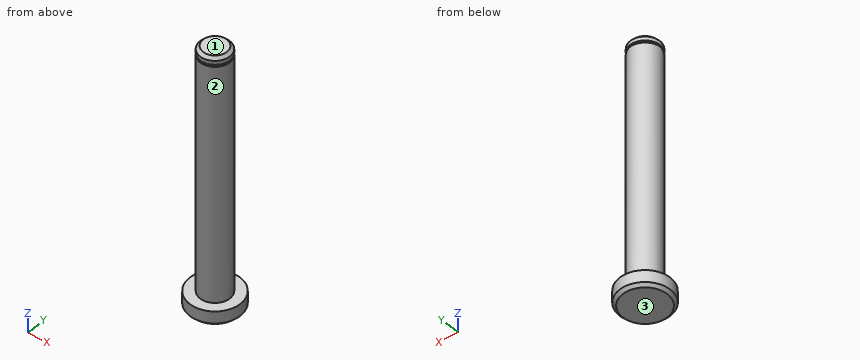
```python
from build123d import *

# Parameters (mm, degrees)
SKETCH1_R               = 8.5
BOSS_EXTRUDE1_DEPTH     = 5
SKETCH2_R               = 5
BOSS_EXTRUDE2_DEPTH     = 82
CHAMFER1_SIZE           = 1
SKETCH3_R               = 14.7
SKETCH3_R_2             = 4.7
CUT_EXTRUDE_THIN1_DEPTH = 0.7


with BuildPart() as part:
    # Sketch1 → Boss-Extrude1 (new body)
    with BuildSketch(Plane.XY):
        Circle(SKETCH1_R)
    extrude(amount=BOSS_EXTRUDE1_DEPTH)

    # Sketch2 → Boss-Extrude2 (add)
    with BuildSketch(Plane.XY.offset(5)):
        Circle(SKETCH2_R)
    extrude(amount=BOSS_EXTRUDE2_DEPTH)

    # Chamfer1
    chamfer1_edges = [part.edges().sort_by_distance(p)[0] for p in [
        (-8.5, 0, 0),
        (-5, 0, 87),
    ]]
    chamfer(chamfer1_edges, length=CHAMFER1_SIZE)

    # Sketch3 → Cut-Extrude-Thin1 (cut)
    with BuildSketch(Plane.XY.offset(84)):
        Circle(SKETCH3_R)
        Circle(SKETCH3_R_2, mode=Mode.SUBTRACT)
    extrude(amount=CUT_EXTRUDE_THIN1_DEPTH, mode=Mode.SUBTRACT)


solid = part.part
```
Source: CAD feature listing. Evaluate the final solid. Frame: model axes, mm. Face numbers are marked on the shaded views. Round coordinates to 2 decimals unless told otherwise and drop trailing zeros. Loops run counter-clockwise (first coordinate to the right, second up) from the corner with the lowest first, then second, coordinate; pieces in that order, holes last.
1. Contact query for flat-ended pins moving along their axis: pin 1 (1.5 mm diameter, centred on x = 1, z = 32, fed in from -Y); pin 2 (1 mm diameter, centred on y = 3, z = 23.5, fed in from +X); pin 3 (5 mm diameter, centred on x = -4, z = 56.5, fed in from +Y). Output: stop coordinate, or through.
2. Ray query, L1, parallel to Z at x = 1.5, y = -7; L2, parallel to Y at x = 1.75, z = 23; L3, parallel to X at y = 0.75, z = 38. Return the intervals inside material, ascending.
3. Section query A-A on x = 0. Output: boundary loops of the cut face in (y, z), and give its area (3 significant figures).
4. Section query C-C on z = 62. Output: boundary loops of the cut face in (x, y), and give its area (3 significant figures).
5. Mould query, pull axis Z, two halves, no side actions, for the marked faces 1, 2 and 3. Classes: released by +Z, released by -Z, zero draft, split by the parting line, or undercut.
Answers below:
1. pin 1: stops at y = -4.99
1. pin 2: stops at x = 4.33
1. pin 3: stops at y = 4.77
2. L1: z = 0 to 5
2. L2: y = -4.68 to 4.68
2. L3: x = -4.94 to 4.94
3. outline: (-8.5, 1) - (-7.5, 0) - (7.5, 0) - (8.5, 1) - (8.5, 5) - (5, 5) - (5, 84) - (4.7, 84) - (4.7, 84.7) - (5, 84.7) - (5, 86) - (4, 87) - (-4, 87) - (-5, 86) - (-5, 84.7) - (-4.7, 84.7) - (-4.7, 84) - (-5, 84) - (-5, 5) - (-8.5, 5) - close
3. area: 903 mm2
4. outline: circle Ø10 at (0, 0)
4. area: 78.5 mm2
5. face 1: released by +Z
5. face 2: zero draft
5. face 3: released by -Z
